Autodesk Inventor part; units mm, degrees
ref_plane "YZ Plane" through (0, 0, 0) normal (1, 0, 0) x (0, 1, 0)
ref_plane "XZ Plane" through (0, 0, 0) normal (0, 1, 0) x (-1, 0, 0)
ref_plane "XY Plane" through (0, 0, 0) normal (0, 0, 1) x (1, 0, 0)
sketch "Sketch1" plane through (0, 0, 0) normal (1, 0, 0) x (0, 1, 0)
  line L0 (0, 0) -> (76.2, 0)
  line L1 (76.2, 0) -> (76.2, -88.9)
  line L2 (76.2, -88.9) -> (0, -88.9)
  line L3 (0, -88.9) -> (0, 0)
  dimension "d0" = 76.2
  dimension "d1" = 88.9
extrude "Extrusion1" add sketch "Sketch1" along normal blind 25.4
sketch "Sketch2" plane through (25.4, 0, 0) normal (1, 0, 0) x (0, 0, -1)
  line L0 (88.9, 76.2) -> (0, 76.2)
  line L1 (44.45, 76.2) -> (44.45, 0)
  line L2 (0, 0) -> (88.9, 0)
  circle A0 centre (44.45, 38.1) radius 14.2875
  line L3 (44.45, 38.1) -> (3.7084, 38.1)
  circle A1 centre (3.7084, 52.832) radius 2.0193
  circle A2 centre (3.7084, 23.368) radius 2.0193
  circle A3 centre (85.1916, 52.832) radius 2.0193
  circle A4 centre (85.1916, 23.368) radius 2.0193
  line L4 (44.45, 38.1) -> (44.45, 68.0212)
  circle A5 centre (44.45, 68.0212) radius 3.302
  circle A6 centre (44.45, 8.1788) radius 3.302
  point P0 (85.1916, 38.1)
  dimension "d4" = 28.575
  dimension "d5" = 40.7416
  dimension "d8" = 29.9212
  dimension "d9" = 6.604
extrude "Extrusion2" cut sketch "Sketch2" against normal up to surface (25.4 mm away)
sketch "Sketch3" plane through (0, 76.2, 0) normal (0, 1, 0) x (1, 0, 0)
  line L0 (0, 88.9) -> (0, 0)
  line L1 (0, 0) -> (25.4, 0)
  line L2 (25.4, 88.9) -> (25.4, 0)
  line L3 (0, 88.9) -> (25.4, 88.9)
extrude "Extrusion3" add sketch "Sketch3" along normal blind 381
chamfer "Chamfer1" distance 38.1 angle 45 1 edges at (12.7, 457.2, 0)
properties part number "launcherV2"
CAD build for the part. Positions are in the model's coordinates, mm. Give positions to 0.01 mm unless a question says otherwise; leave off trailing zeros. Order: outer loops, then holes, each group sorted by start corner. A loop starts at its lowest first (then second) coordinate and runs counter-clockwise, first axis right, second up.
(1) Saw through at B-B, the plane z = -54.5. Give the cut face in (x, y), then the cut area to 3 significant figures.
(2) Drill centre lines: L1, parallel to Y at x = 9.75, z = -44.45; L2, parallel to Y at x = 18, z = -84; L3, parallel to Y at x = 14, z = -85. Where is each one in solid material? Low to high.
(3) Mould opens along Y. For faces 1 (the cylindrical face through (12.88, 29.41, -33.11)), 2 (the flat face through (12.5, 437.9, -18.8)), 3 (the flat face through (25.4, 225, -45)), 4 (the flat face through (13, 0, -45)) say: released by +Y, released by -Y, zero draft, split by the parting line, or undercut.
(4) Flat gauge pins, fed straight in: pin 1 (2.5 mm diameter, centred on y = 52.83, z = -85.19, fed in from +X); pin 2 (4 mm diameter, centred on x = 17, z = -35.5, fed in from +Y). Where does each tip first touch, or does it go through?
(5) Saw through at C-C, the plane x = 3.75. State how many separate pieces and enclosed holes the cut face has, then the cut area to 3 significant figures.
(6) Saw through at A-A, the plane y = 38.1. Give the cut face in (x, z).
Results found:
1. outline: (0, 0) - (25.4, 0) - (25.4, 27.94) - (0, 27.94) - close; (0, 48.26) - (25.4, 48.26) - (25.4, 457.2) - (0, 457.2) - close
1. area: 11,100 mm2
2. L1: y = 0 to 4.88, 11.48 to 23.81, 52.39 to 64.72, 71.32 to 457.2
2. L2: y = 0 to 21.74, 25 to 51.2, 54.46 to 457.2
2. L3: y = 0 to 21.36, 25.38 to 50.82, 54.84 to 457.2
3. face 1: undercut
3. face 2: released by +Y
3. face 3: zero draft
3. face 4: released by -Y
4. pin 1: passes through
4. pin 2: stops at y = 456.6
5. separate pieces: 1
5. enclosed holes: 7
5. area: 39,200 mm2
6. outline: (0, -88.9) - (25.4, -88.9) - (25.4, -58.74) - (0, -58.74) - close; (0, -30.16) - (25.4, -30.16) - (25.4, 0) - (0, 0) - close
